from build123d import *

# Parameters (mm, degrees)
ESBO_O1_W                = 150
ESBO_O1_H                = 100
RESSALTO_EXTRUS_O1_DEPTH = 6
ESBO_O3_W                = 6
ESBO_O3_H                = 30
RESSALTO_EXTRUS_O2_DEPTH = 6
ESBO_O4_W                = 6
ESBO_O4_H                = 30
RESSALTO_EXTRUS_O3_DEPTH = 6
ESBO_O6_W                = 6
ESBO_O6_H                = 36
RESSALTO_EXTRUS_O4_DEPTH = 6
ESBO_O7_W                = 6
ESBO_O7_H                = 36
RESSALTO_EXTRUS_O5_DEPTH = 6
ESBO_O8_W                = 162
ESBO_O8_H                = 5.982470976
CORTE_EXTRUS_O1_DEPTH    = 6


with BuildPart() as part:
    # Esboço1 → Ressalto-extrusão1 (new body)
    with BuildSketch(Plane(origin=(0, 0, 0), x_dir=(0, 0, -1), z_dir=(1, 0, 0))):
        Rectangle(ESBO_O1_W, ESBO_O1_H)
    extrude(amount=RESSALTO_EXTRUS_O1_DEPTH)

    # Esboço3 → Ressalto-extrusão2 (add)
    with BuildSketch(Plane(origin=(0, 50, 0), x_dir=(1, 0, 0), z_dir=(0, 1, 0))):
        with Locations((3, 60)):
            Rectangle(ESBO_O3_W, ESBO_O3_H)
        with Locations((3, 0)):
            Rectangle(ESBO_O3_W, ESBO_O3_H)
        with Locations((3, -60)):
            Rectangle(ESBO_O3_W, ESBO_O3_H)
    extrude(amount=RESSALTO_EXTRUS_O2_DEPTH)

    # Esboço4 → Ressalto-extrusão3 (add)
    with BuildSketch(Plane.XZ.offset(50)):
        with Locations((3, 60)):
            Rectangle(ESBO_O4_W, ESBO_O4_H)
        with Locations((3, 0)):
            Rectangle(ESBO_O4_W, ESBO_O4_H)
        with Locations((3, -60)):
            Rectangle(ESBO_O4_W, ESBO_O4_H)
    extrude(amount=RESSALTO_EXTRUS_O3_DEPTH)

    # Esboço6 → Ressalto-extrusão4 (add)
    with BuildSketch(Plane.XY.offset(75)):
        with Locations((3, 38)):
            Rectangle(ESBO_O6_W, ESBO_O6_H)
        with Locations((3, -38)):
            Rectangle(ESBO_O6_W, ESBO_O6_H)
    extrude(amount=RESSALTO_EXTRUS_O4_DEPTH)

    # Esboço7 → Ressalto-extrusão5 (add)
    with BuildSketch(Plane(origin=(0, 0, -75), x_dir=(-1, 0, 0), z_dir=(0, 0, -1))):
        with Locations((-3, -38)):
            Rectangle(ESBO_O7_W, ESBO_O7_H)
        with Locations((-3, 38)):
            Rectangle(ESBO_O7_W, ESBO_O7_H)
    extrude(amount=RESSALTO_EXTRUS_O5_DEPTH)

    # Esboço8 → Corte-extrusão1 (cut)
    with BuildSketch(Plane.ZY):
        with Locations((0, 53.008764512)):
            Rectangle(ESBO_O8_W, ESBO_O8_H)
    extrude(amount=-CORTE_EXTRUS_O1_DEPTH, mode=Mode.SUBTRACT)


solid = part.part
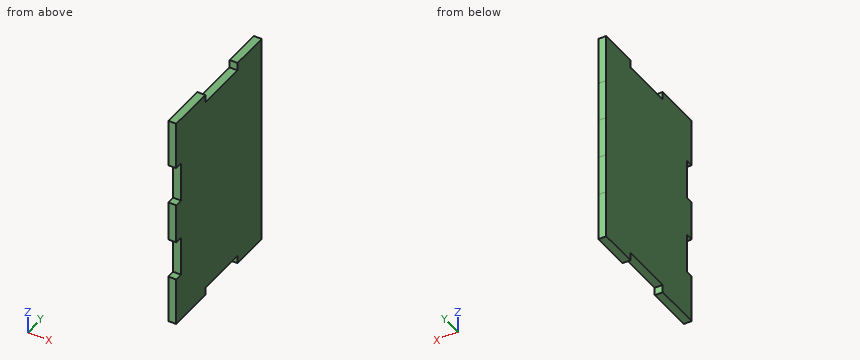
Could you check a few things on this model? Use its own coordinates, in mm. Give positions to 0.01 mm unless a question says otherwise; leave off trailing zeros. Write each loop counter-clockwise with the first axis right and the second up, starting at its lowest first coordinate (ties: lowest second). Pieces come first, ordered by that corner, then holes. Notation, with made-up numbers: (26, -22) -> (66, -22) arc R22 cw to (66, 0) -> close; hole circle Ø1 at (9.25, -39). An arc over 180 degrees is marked (long way). Answer as a JSON object with one key per item and string values.
Q1. Will these pins go through, and if not, where does the flat tip stop? pin 1 Ø1.8 at (x, y) = (4.5, -9.5) entering from +Z; pin 2 Ø3 at (x, z) = (3.5, -36) entering from +Y; pin 3 Ø1.8 at (x, y) = (3.5, -9) entering from -Z.
Taken from the geometry:
{"pin 1": "stops at z = 75", "pin 2": "stops at y = 50", "pin 3": "stops at z = -75"}
Q2. Suppose I cut it at B-B on y = -4. Write out the boundary of the cut face in (x, z), then the cut area to 3 significant figures.
Taken from the geometry:
{"outline": "(0, -75) -> (6, -75) -> (6, 75) -> (0, 75) -> close", "area": "900 mm²"}
Q3. Please list where these lines run through material, in increasing order: L1, parallel to Y at x = 2.9, z = -34; L2, parallel to Z at x = 3.55, y = 12.
Taken from the geometry:
{"L1": "y = -50 to 50", "L2": "z = -75 to 75"}
Q4. Suppose I cut it at C-C on z = -37. Write out the boundary of the cut face in (x, y).
Taken from the geometry:
{"outline": "(0, -50) -> (6, -50) -> (6, 50) -> (0, 50) -> close"}
